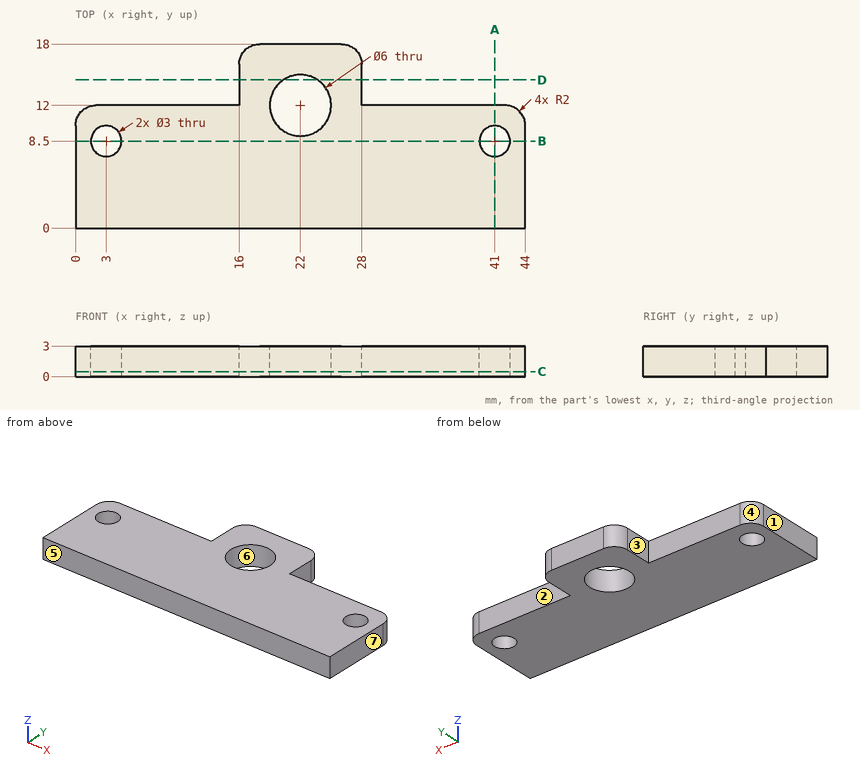
Job drawing, mm, ordinate dimensions from the low corner. One solid piece. A direction names the side the tool comes from. Give positions to 0.01 mm unless a question says otherwise; leave off trailing zeros. Write each loop counter-clockwise with the first axis right and the second up, starting at its lowest first coordinate (ties: lowest second). Pieces come first, ordered by that corner, then holes. Notation, with made-up numbers: (86, -32) - (121, -32) arc R19 cw to (121, -5) - close; hole circle Ø6 at (-25.75, 52.25). An arc over 180 degrees is marked (long way). Use one line per item in the form item = value. Start each with the question number.
1. Probe line 1 (X direction, y = 8.5, z = 2.1); line 2 (Y direction, x = 22, z = 0.85); line 3 (Y direction, x = 41, z = 1.3). List the from-to ranges inside material, lowest first. Write a range as [from, to].
2. Band-saw the part on B-B on y = 8.5. Write the cut outline in (x, z), plus the area to 3 significant figures.
3. Band-saw the part on C-C on z = 0.5. Write the cut outline in (x, y).
4. Two-plate mould, pull along Y, no slides. Class the marked faces 4, 5, 6 and 7: released by +Y, released by -Y, zero draft, split by the parting line, or undercut.
5. Band-saw the part on D-D on y = 14.5. Write the cut outline in (x, z).
6. Drop a flat-ended pin along its axis: pin 1 Ø10 at (x, y) = (16, 15.5) entering from -Z. Give the stop position or say it passes through.
7. 3-axis set-ups, long thin cutter, end or side, ignore diameter. For the marked faces 1, 2 and 3: which of +Z, -Z, +X, -X, +Y, -Y reach the whole face in a straight line?
8. Band-saw the part on A-A on x = 41. Write the cut outline in (y, z), plus the area to 3 significant figures.
Conclusion:
q1.line_1 = [0, 1.5], [4.5, 39.5], [42.5, 44]
q1.line_2 = [0, 9], [15, 18]
q1.line_3 = [0, 7], [10, 12]
q2.outline = (0, 0) - (1.5, 0) - (1.5, 3) - (0, 3) - close; (4.5, 0) - (39.5, 0) - (39.5, 3) - (4.5, 3) - close; (42.5, 0) - (44, 0) - (44, 3) - (42.5, 3) - close
q2.area = 114 mm²
q3.outline = (0, 0) - (44, 0) - (44, 10) arc R2 ccw to (42, 12) - (28, 12) - (28, 16) arc R2 ccw to (26, 18) - (18, 18) arc R2 ccw to (16, 16) - (16, 12) - (2, 12) arc R2 ccw to (0, 10) - close; hole circle Ø3 at (3, 8.5); hole circle Ø6 at (22, 12); hole circle Ø3 at (41, 8.5)
q4.face_4 = released by +Y
q4.face_5 = released by -Y
q4.face_6 = undercut
q4.face_7 = zero draft
q5.outline = (16, 0) - (20.34, 0) - (20.34, 3) - (16, 3) - close; (23.66, 0) - (28, 0) - (28, 3) - (23.66, 3) - close
q6.pin_1 = 0
q7.face_1 = +Z, -Z, -X, +Y, -Y
q7.face_2 = +Z, -Z, +X, +Y
q7.face_3 = +Z, -Z, -X, +Y
q8.outline = (0, 0) - (7, 0) - (7, 3) - (0, 3) - close; (10, 0) - (12, 0) - (12, 3) - (10, 3) - close
q8.area = 27.0 mm²
